Verification items for the finished model (mm, model axes). Face numbers are marked on the shaded views. A direction names the side the tool comes from. Give positions to 0.01 mm unless a question says otherwise; leave off trailing zeros. Order: outer loops, then holes, each group sorted by start corner. A loop starts at its lowest first (then second) coordinate and runs counter-clockwise, first axis right, second up. Notation, with made-up numbers: M 43,21 L 86,21 A36 cw 86,57 Z; hole C -28,86 d3. An arc over 180 degrees is marked long. Answer as a JSON object with one key per item and string values.
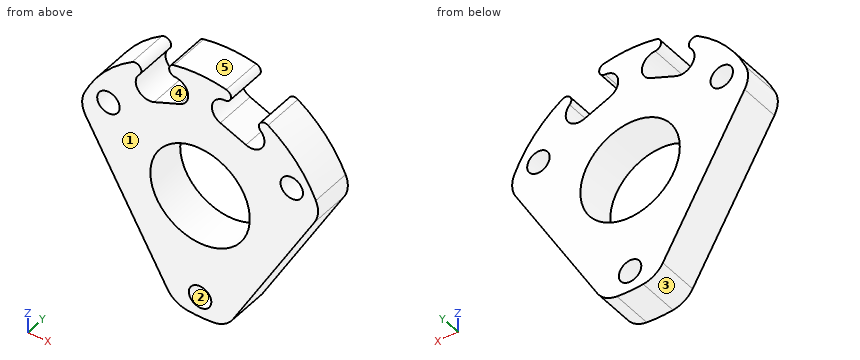
Autodesk Inventor part; units mm, degrees
ref_plane "YZ Plane" through (0, 0, 0) normal (1, 0, 0) x (0, 1, 0)
ref_plane "XZ Plane" through (0, 0, 0) normal (0, 1, 0) x (-1, 0, 0)
ref_plane "XY Plane" through (0, 0, 0) normal (0, 0, 1) x (1, 0, 0)
sketch "Sketch1" plane through (0, 0, 0) normal (0, 1, 0) x (-1, 0, 0)
  circle A0 centre (-0.0038, -16.5528) radius 1.75
  circle A1 centre (-0.0038, -0.0528) radius 7.75
  circle A2 centre (-14.2932, 8.1972) radius 1.75
  circle A3 centre (14.2856, 8.1972) radius 1.75
  arc A4 (3.9019, 17.421) -> (3.1441, 13.3853) centre (3.9353, 15.3257) ccw
  arc A5 (3.9019, 17.421) -> (4.0803, 19.2703) centre (3.8869, 18.3557) ccw
  arc A6 (4.0803, 19.2703) -> (-4.0878, 19.2703) centre (-0.0038, -0.0528) ccw
  arc A7 (-4.0878, 19.2703) -> (-3.9094, 17.421) centre (-3.8945, 18.3557) ccw
  arc A8 (-3.1517, 13.3853) -> (-3.9094, 17.421) centre (-3.9429, 15.3257) ccw
  line L0 (-3.1517, 13.3853) -> (-7.1501, 11.755)
  arc A9 (-9.4303, 15.1698) -> (-7.1501, 11.755) centre (-7.9413, 13.6954) ccw
  arc A10 (-9.4303, 15.1698) -> (-10.596, 16.6166) centre (-10.0946, 15.8276) ccw
  arc A11 (-10.596, 16.6166) -> (-18.0415, 7.991) centre (-0.0038, -0.0528) ccw
  arc A12 (-18.0415, 7.991) -> (-17.8524, 4.3619) centre (-14.3883, 6.3619) ccw
  line L1 (-17.8524, 4.3619) -> (-5.1048, -17.7175)
  arc A13 (-5.1048, -17.7175) -> (-2.0565, -19.6958) centre (-1.6407, -15.7175) ccw
  arc A14 (-2.0565, -19.6958) -> (2.0489, -19.6958) centre (-0.0038, -0.0528) ccw
  arc A15 (2.0489, -19.6958) -> (5.0973, -17.7175) centre (1.6332, -15.7175) ccw
  line L2 (5.0973, -17.7175) -> (17.8448, 4.3619)
  arc A16 (17.8448, 4.3619) -> (18.0339, 7.991) centre (14.3807, 6.3619) ccw
  arc A17 (18.0339, 7.991) -> (10.5884, 16.6166) centre (-0.0038, -0.0528) ccw
  arc A18 (10.5884, 16.6166) -> (9.4227, 15.1698) centre (10.087, 15.8276) ccw
  arc A19 (7.1425, 11.755) -> (9.4227, 15.1698) centre (7.9337, 13.6954) ccw
  line L3 (7.1425, 11.755) -> (3.1441, 13.3853)
extrude "Extrusion1" add sketch "Sketch1" along normal blind 6.35
properties part number "LowerPlate"
Q1. Tool access check on the marked faces 4 and 5. Record the directions out of +Z, -Z, +X, -X, +Y, -Y that give a thin tool (end or side, any length) a straight path to the whole face; none if there is none.
Resolved:
{"face 4": "+Y, -Y", "face 5": "+Z, +Y, -Y"}
Q2. Section check D-D on y = 2. Count the separate pieces of the cut face and the enclosed holes in it, then the cut area to 3 significant figures.
Resolved:
{"separate pieces": "1", "enclosed holes": "4", "area": "659 mm²"}
Q3. Material ranges on L1, parallel to X at y = 5.75, z = 9; L2, parallel to X at y = 2.5, z = 3; L3, parallel to X at y = 4, z = 0.5, recorded low to high.
Resolved:
{"L1": "x = -17.55 to -15.84, -12.73 to 12.74, 15.85 to 17.56", "L2": "x = -17.06 to -7.12, 7.13 to 17.07", "L3": "x = -15.62 to -7.73, 7.73 to 15.62"}
Q4. Gauge pin test, flat end, axial feed: pin 1 Ø1.5 at (y, z) = (3.5, -8.5) entering from +X. Record the tip position at first contact, or that the pin passes through.
Resolved:
{"pin 1": "stops at x = 10.86"}
Q5. Section check B-B on x = -13. Record the cut outline in (y, z).
Resolved:
{"outline": "M 0,-4.03 L 6.35,-4.03 L 6.35,7.01 L 0,7.01 Z; M 0,9.38 L 6.35,9.38 L 6.35,14.81 L 0,14.81 Z"}
Q6. Section check C-C on x = 1. Record the cut outline in (y, z).
Resolved:
{"outline": "M 0,-19.78 L 6.35,-19.78 L 6.35,-17.99 L 0,-17.99 Z; M 0,-15.11 L 6.35,-15.11 L 6.35,-7.74 L 0,-7.74 Z; M 0,7.63 L 6.35,7.63 L 6.35,19.67 L 0,19.67 Z"}
Q7. Release check for a two-part mould opening along X. For the marked faces 1, 2 and 3 record: +X half, -X half, draft (parallel to the pull), parting line (faces both ways), or undercut.
Resolved:
{"face 1": "draft", "face 2": "undercut", "face 3": "-X half"}
Q8. Section check A-A on z = 9. Record the cut outline in (x, y).
Resolved:
{"outline": "M -17.55,0 L -15.84,0 L -15.84,6.35 L -17.55,6.35 Z; M -12.73,0 L 12.74,0 L 12.74,6.35 L -12.73,6.35 Z; M 15.85,0 L 17.56,0 L 17.56,6.35 L 15.85,6.35 Z"}
